Check sheet for the modelled part. Datum: model origin and axes. Units: mm. Face numbers are marked on the shaded views. A direction names the side the tool comes from. Give positions to 0.01 mm unless a question says otherwise; leave off trailing zeros. Loops run counter-clockwise (first coordinate to the right, second up) from the corner with the lowest first, then second, coordinate; pieces in that order, holes last. Notation, with made-up numbers: M 60,-27 L 68,-27 A20 ccw 68,-8 Z; hole C 47.25,84.25 d2. An arc over 180 degrees is marked long. One line per question, with ' | ' between items. Start each with the question number.
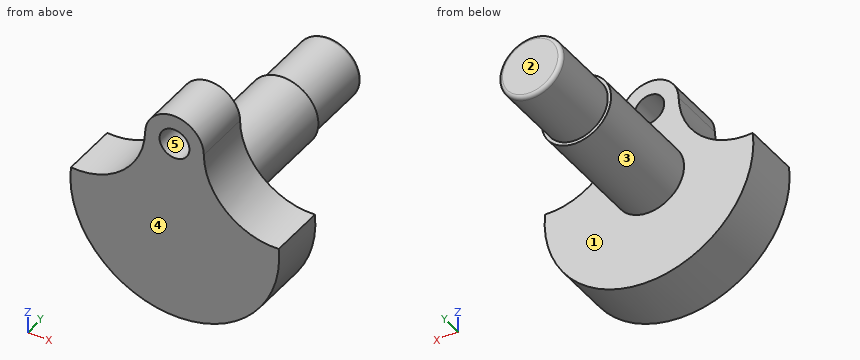
from build123d import *

# Parameters (mm, degrees)
F0_R     = 3.0099
F1_DEPTH = 11.43
F2_R     = 6.9977
F2_R_2   = 6.3373
F3_DEPTH = 23.0124
F4_DEPTH = 37.5666
F5_R     = 0.762


with BuildPart() as f1:
    # F0 (on Front) → F1 (new body)
    with BuildSketch(Plane.XZ):
        with BuildLine():
            ThreePointArc((20.977623, 1.152295), (10.42378, 4.807532), (5.905392, 15.021665))
            ThreePointArc((5.905392, 15.021665), (0.041118, 20.891357), (-5.904323, 15.103895))
            ThreePointArc((-5.904323, 15.103895), (-10.442291, 5.064331), (-20.839523, 1.41967))
            ThreePointArc((-20.839523, 1.41967), (-0.078135, -21.733629), (20.977623, 1.152295))
        make_face()
        with Locations((0, 14.986)):
            Circle(F0_R, mode=Mode.SUBTRACT)
    extrude(amount=F1_DEPTH)

    # F2 (on Front) → F3 (join)
    with BuildSketch(Plane.XZ):
        Circle(F2_R)
        Circle(F2_R_2, mode=Mode.SUBTRACT)
    extrude(amount=-F3_DEPTH)

    # F2 (on Front) → F4 (join)
    with BuildSketch(Plane.XZ):
        Circle(F2_R_2)
    extrude(amount=-F4_DEPTH)

    # F5
    f5_edges = [f1.edges().sort_by_distance(p)[0] for p in [
        (-6.3373, 37.5666, 0),
    ]]
    fillet(f5_edges, radius=F5_R)


solid = f1.part
Q1. Access from +Z, -Z, +X, -X, +Y, -Y to the whole of each face (thin tool, end or side, straight path). Record for the marked faces 1 and 2.
Q2. Cross-section at C-C (y = -3.5). Record the cut outline in (x, z).
Q3. Draft check along X on the marked faces 3, 4 and 5. Enter one of: released by +X, released by -X, zero draft, split by the parting line, or undercut.
Q4. Cross-section at B-B (x = 0). Record the cut outline in (y, z).
Q5. Depth check by flat-ended pin: P1, Ø6, axis at x = -11.5, y = 27.5, coming from the +Z side; P2, Ø12, axis at x = 2.5, y = 5.5, coming from the -Z side; P3, Ø12, axis at x = -7, y = 28, coming from the +Z side; P4, Ø10, axis at y = 4, z = 11.5, coming from the +X side. Enter the tip coordinate at first touch or a pass-through.
Q6. Cross-section at D-D (z = 0). Record the cut outline in (x, y), and give its area (3 significant figures).
Q7. Cross-section at A-A (z = 16.5). Record the cut outline in (x, y).
Q8. Material ranges on probe 1 along Z at (x, y) = (0, -5.5); probe 2 along Y at (x, z) = (-4, -6.5); probe 3 along X at (y, z) = (1, 2.5), recorded low to high. Write a range as from..to.
Solved:
1) face 1: +Y | face 2: +Z, -Z, +X, -X, +Y
2) outline: M -20.84,1.42 A21.01 ccw long 20.98,1.15 A14 cw 5.91,15.02 A5.91 ccw -5.9,15.1 A14 cw Z; hole C 0,14.99 d6.02
3) face 3: split by the parting line | face 4: zero draft | face 5: undercut
4) outline: M -11.43,-21.73 L 0,-21.73 L 0,-7 L 23.01,-7 L 23.01,-6.34 L 36.8,-6.34 A0.76 ccw 37.57,-5.58 L 37.57,5.58 A0.76 ccw 36.8,6.34 L 23.01,6.34 L 23.01,7 L 0,7 L 0,11.98 L -11.43,11.98 Z; M -11.43,18 L 0,18 L 0,20.89 L -11.43,20.89 Z
5) P1: passes through | P2: stops at z = -21.73 | P3: stops at z = 6.26 | P4: stops at x = 7.56
6) outline: M -20.94,-11.43 L 21.05,-11.43 L 21.05,0 L 7,0 L 7,23.01 L 6.34,23.01 L 6.34,36.8 A0.76 ccw 5.58,37.57 L -5.58,37.57 A0.76 ccw -6.34,36.8 L -6.34,23.01 L -7,23.01 L -7,0 L -20.94,0 Z | area: 986 mm²
7) outline: M -5.71,-11.43 L -2.6,-11.43 L -2.6,0 L -5.71,0 Z; M 2.6,-11.43 L 5.71,-11.43 L 5.71,0 L 2.6,0 Z
8) probe 1: z = -21.73..11.98, 18..20.89 | probe 2: y = -11.43..0 | probe 3: x = -6.54..6.54
